Source: CAD feature listing. Evaluate the final solid. Frame: model axes, mm. Face numbers are marked on the shaded views. A direction names the side the tool comes from. Give positions to 0.01 mm unless a question says otherwise; leave off trailing zeros. Order: outer loops, then holes, each group sorted by start corner. A loop starts at its lowest first (then second) coordinate and runs counter-clockwise, first axis right, second up. Notation, with made-up numbers: (-28.75, 8) - (9.25, 8) arc R14 ccw to (9.25, 15) - close; hole circle Ø3 at (-39, -2). An arc over 180 degrees is marked (long way). Write each question's results on one line, items separated by ' | '. Start each with the question number.
Item 1: Mould query, pull axis X, two halves, no side actions, for the marked faces 1, 2 and 3. Classes: released by +X, released by -X, zero draft, split by the parting line, or undercut.
Item 2: Section B-B on x = 28.25. Output: boundary loops of the cut face in (y, z).
Item 3: Section D-D on z = 0.75. Output: boundary loops of the cut face in (x, y).
Item 4: Section A-A on y = -1.25. Output: boundary loops of the cut face in (x, z).
Item 5: Section C-C on x = 25.5. Output: boundary loops of the cut face in (y, z), and give its area (3 significant figures).
Item 6: Line query: line 1 along X through (y, z) = (0.5, 0.5); line 2 along Y through (x, z) = (25.5, 5.75); line 3 along Z through (x, y) = (20.5, 1). Output: solid intervals per line, ascending.
Item 7: Contact query for flat-ended pins moving along their axis: pin 1 Ø5 at (x, y) = (24.5, 3.5) entering from +Z; pin 2 Ø3 at (x, y) = (13.5, -3.5) entering from -Z; pin 3 Ø8 at (x, z) = (27.5, 6.5) entering from +Y; pin 4 Ø1.8 at (x, y) = (12.61, 0.6) entering from -Z. Output: stop coordinate, or through.
Item 8: Set-up query: the marked faces 4, 5 and 6. Return all of +Z, -Z, +X, -X, +Y, -Y with unobstructed straight access to the full face (end or side cutting, diameter ignored); none if empty.
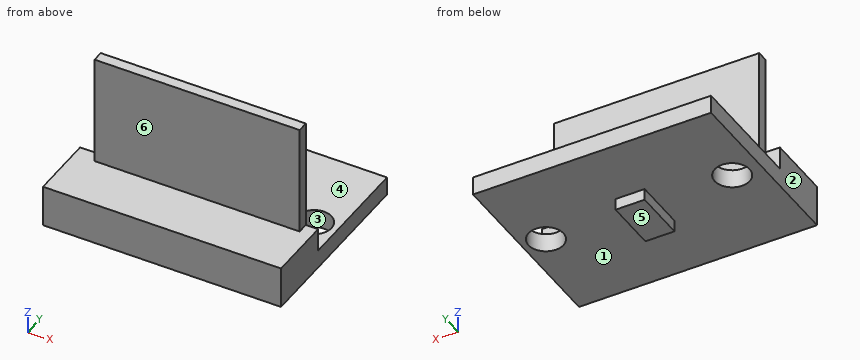
Autodesk Inventor part; units mm, degrees
ref_plane "YZ Plane" through (0, 0, 0) normal (1, 0, 0) x (0, 1, 0)
ref_plane "XZ Plane" through (0, 0, 0) normal (0, 1, 0) x (-1, 0, 0)
ref_plane "XY Plane" through (0, 0, 0) normal (0, 0, 1) x (1, 0, 0)
sketch "Boceto1" plane through (0, 0, 0) normal (0, 0, 1) x (1, 0, 0)
  circle A0 centre (20.3885, 0.1002) radius 16.5
  circle A1 centre (20.3885, 0.1002) radius 19.85
  line L0 (10.1635, 8.1002) -> (30.6135, 8.1002)
  line L1 (30.6135, 8.1002) -> (30.6135, -7.8998)
  line L2 (30.6135, -7.8998) -> (10.1635, -7.8998)
  line L3 (10.1635, -7.8998) -> (10.1635, 8.1002)
  line L4 (10.1635, 8.1002) -> (30.6135, -7.8998) construction
  line L5 (30.6135, 8.1002) -> (10.1635, -7.8998) construction
  point P0 (0, 0)
  dimension "d0" = 20.45
  dimension "d1" = 16
extrude "Extrusión1" add sketch "Boceto1" along normal blind 1.6 contours L0 L1 L2 L3
sketch "Boceto2" plane through (0, 0, 1.6) normal (0, 0, 1) x (1, 0, 0)
  line L0 (10.1635, -7.8998) -> (30.6135, -7.8998)
  line L1 (30.6135, -7.8998) -> (30.6135, -2.2998)
  line L2 (30.6135, -7.8998) -> (30.6135, 8.1002)
  line L3 (30.6135, -2.2998) -> (10.1635, -2.2998)
  line L4 (10.1635, 8.1002) -> (10.1635, -7.8998)
  line L5 (10.1635, -7.8998) -> (10.1635, -2.2998)
  line L6 (30.6135, -7.8998) -> (10.1635, -7.8998)
  point P0 (0, 0)
  dimension "d4" = 5.6
extrude "Extrusión2" add sketch "Boceto2" along normal blind 11.5
sketch "Boceto3" plane through (0, 0, 13.1) normal (0, 0, 1) x (1, 0, 0)
  line L0 (30.6135, -2.2998) -> (10.1635, -2.2998)
  line L1 (11.9387, -2.2998) -> (10.1635, -2.2998)
  line L2 (10.1635, -2.2998) -> (10.1635, -7.8194)
  line L3 (10.1635, -7.8194) -> (30.6135, -7.8194)
  line L4 (30.6135, -7.8194) -> (30.6135, -2.2998)
  line L5 (30.6135, -2.2998) -> (29.5577, -2.2998)
  line L6 (29.5577, -3.2351) -> (11.9387, -3.2351)
  line L7 (11.9387, -3.2351) -> (11.9387, -2.2998)
  line L8 (29.5577, -2.2998) -> (29.5577, -3.2351)
  point P0 (0, 0)
extrude "Extrusión3" cut sketch "Boceto3" against normal blind 9.5 contours L4 L3 L2 L0 L7 L6 L8
sketch "Boceto4" plane through (0, 0, 13.1) normal (0, 0, 1) x (1, 0, 0)
  line L0 (30.6135, -7.8194) -> (10.1635, -7.8194)
  line L1 (10.1635, -7.8194) -> (10.1635, -7.8998)
  line L2 (10.1635, -7.8998) -> (30.6135, -7.8998)
  line L3 (30.6135, -7.8998) -> (30.6135, -7.8194)
  point P0 (0, 0)
extrude "Extrusión4" cut sketch "Boceto4" against normal blind 9.5
sketch "Boceto5" plane through (0, 0, 1.6) normal (0, 0, 1) x (1, 0, 0)
  circle A0 centre (28.6135, 0.6002) radius 1.5
  line L0 (28.6135, 0.6002) -> (12.6135, 0.6002) construction
  line L1 (28.6135, 0.6002) -> (44.6135, 0.6002) construction
  circle A1 centre (12.6135, 0.6002) radius 1.5
  point P0 (0, 0)
  point P1 (30.6135, 8.1002)
  dimension "d14" = 16
  dimension "d15" = 180
  dimension "d16" = 3
extrude "Extrusión5" cut sketch "Boceto5" against normal through all
sketch "Boceto6" plane through (0, 0, 0) normal (0, 0, -1) x (-1, 0, 0)
  line L0 (-10.1635, -7.8998) -> (-10.1635, 8.1002) construction
  line L1 (-30.6135, -7.8998) -> (-10.1635, -7.8998) construction
  line L2 (-10.1635, 8.1002) -> (-30.6135, -7.8998) construction
  line L3 (-30.6135, 8.1002) -> (-30.6135, -7.8998) construction
  line L4 (-10.1635, -7.8998) -> (-30.6135, 8.1002) construction
  line L5 (-19.1385, 2.3502) -> (-21.6385, 2.3502)
  line L6 (-21.6385, 2.3502) -> (-21.6385, -2.1498)
  line L7 (-21.6385, -2.1498) -> (-19.1385, -2.1498)
  line L8 (-19.1385, -2.1498) -> (-19.1385, 2.3502)
  line L9 (-19.1385, 2.3502) -> (-21.6385, -2.1498) construction
  line L10 (-21.6385, 2.3502) -> (-19.1385, -2.1498) construction
  point P0 (0, 0)
  point P1 (-20.3885, 0.1002)
  dimension "d19" = 2.5
  dimension "d20" = 4.5
extrude "Extrusión6" add sketch "Boceto6" along normal blind 1
properties part number "SensorCJMCU530"
Evaluation:
1) face 1: zero draft | face 2: released by -X | face 3: undercut
2) outline: (-7.9, 0) - (-0.86, 0) - (-0.86, 1.6) - (-2.3, 1.6) - (-2.3, 13.1) - (-3.24, 13.1) - (-3.24, 3.6) - (-7.9, 3.6) - close; (2.06, 0) - (8.1, 0) - (8.1, 1.6) - (2.06, 1.6) - close
3) outline: (10.16, -7.9) - (30.61, -7.9) - (30.61, 8.1) - (10.16, 8.1) - close; hole circle Ø3 at (12.61, 0.6); hole circle Ø3 at (28.61, 0.6)
4) outline: (10.16, 0) - (19.14, 0) - (19.14, -1) - (21.64, -1) - (21.64, 0) - (30.61, 0) - (30.61, 1.6) - (10.16, 1.6) - close
5) outline: (-7.9, 0) - (8.1, 0) - (8.1, 1.6) - (-2.3, 1.6) - (-2.3, 13.1) - (-3.24, 13.1) - (-3.24, 3.6) - (-7.9, 3.6) - close | area: 45.7 mm^2
6) line 1: x = 10.16 to 11.12, 14.11 to 27.12, 30.11 to 30.61 | line 2: y = -3.24 to -2.3 | line 3: z = -1 to 1.6
7) pin 1: stops at z = 1.6 | pin 2: stops at z = 0 | pin 3: stops at y = -2.3 | pin 4: passes through
8) face 4: +Z, +X, -X, +Y | face 5: -Z, +X, -X, +Y, -Y | face 6: +Z, +X, -X, -Y
